Verification items for the finished model (mm, model axes). Face numbers are marked on the shaded views. A direction names the side the tool comes from. Round coordinates to 2 decimals unless told otherwise and drop trailing zeros. Order: outer loops, then holes, each group sorted by start corner. A loop starts at its lowest first (then second) coordinate and runs counter-clockwise, first axis right, second up. Notation, with made-up numbers: (11, 42.25) -> (68, 42.25) arc R32 ccw to (68, 78.25) -> close; hole circle Ø10 at (37.5, 27.25). An arc over 180 degrees is marked (long way). Write item = value, one per line. Start each with the question number.
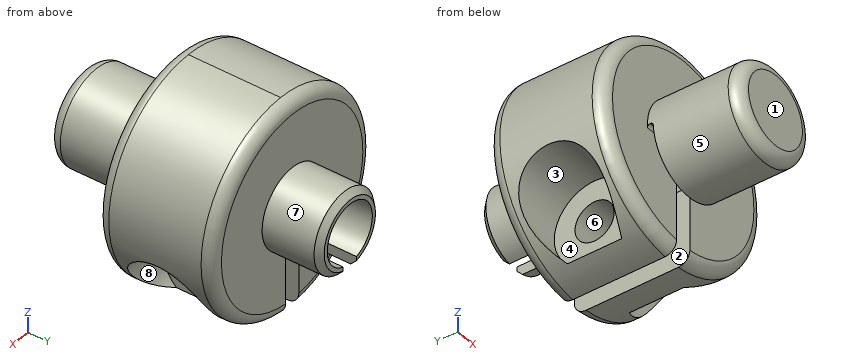
from build123d import *

# Parameters (mm, degrees)
SKETCH1_R            = 4.05
BOSS_EXTRUDE1_DEPTH  = 8
SKETCH2_R            = 9
BOSS_EXTRUDE2_DEPTH  = 10
FILLET1_R            = 1
SKETCH3_R            = 2.55
CUT_EXTRUDE1_DEPTH   = 10
CUT_EXTRUDE2_REACH   = 24.045
M3_CLEARANCE_HOLE1_D = 3.4
SKETCH28_R           = 3.5
CUT_EXTRUDE3_DEPTH   = 6.5
SKETCH29_W           = 8.1
SKETCH29_H           = 0.5
CUT_EXTRUDE7_DEPTH   = 23.045407848
FILLET2_R            = 0.25
BOSS_EXTRUDE3_START  = 5
BOSS_EXTRUDE3_DEPTH  = 5
CHAMFER1_SIZE        = 0.5


with BuildPart() as part:
    # Sketch1 → Boss-Extrude1 (new body)
    with BuildSketch(Plane(origin=(0, 0, 0), x_dir=(1, 0, 0), z_dir=(0, 1, 0))):
        with Locations(Location((0, 0, 0), (0, 0, 270))):
            Circle(SKETCH1_R)
    extrude(amount=BOSS_EXTRUDE1_DEPTH)

    # Sketch2 → Boss-Extrude2 (add)
    with BuildSketch(Plane(origin=(0, 8, 0), x_dir=(1, 0, 0), z_dir=(0, 1, 0))):
        with Locations(Location((0, 0, 0), (0, 0, 270))):
            Circle(SKETCH2_R)
    extrude(amount=BOSS_EXTRUDE2_DEPTH)

    # Fillet1
    fillet1_edges = [part.edges().sort_by_distance(p)[0] for p in [
        (0, 0, -4.05),
        (0, 8, -9),
        (0, 18, -9),
    ]]
    fillet(fillet1_edges, radius=FILLET1_R)

    # Sketch3 → Cut-Extrude1 (cut)
    with BuildSketch(Plane(origin=(0, 18, 0), x_dir=(1, 0, 0), z_dir=(0, 1, 0))):
        with Locations(Location((0, 0, 0), (0, 0, 270))):
            Circle(SKETCH3_R)
    extrude(amount=-CUT_EXTRUDE1_DEPTH, mode=Mode.SUBTRACT)

    # Cut-Extrude2: up to this face of the body (flat: up to its plane)
    cut_extrude2_end = Plane(part.part.faces().sort_by_distance((0, 8, -7.77372583))[0])
    # Sketch20 → Cut-Extrude2 (cut, up to the picked face)
    with BuildSketch(Plane(origin=(0, 18, 0), x_dir=(1, 0, 0), z_dir=(0, 1, 0)), mode=Mode.PRIVATE) as cut_extrude2_sk1:
        with BuildLine():
            Line((-0.75, 2.437211521), (0.75, 2.437211521))
            Line((0.75, 2.437211521), (0.75, 8.968695557))
            ThreePointArc((0.75, 8.968695557), (0, 9), (-0.75, 8.968695557))
            Line((-0.75, 8.968695557), (-0.75, 2.437211521))
        make_face()
    cut_extrude2_tool1 = split(extrude(cut_extrude2_sk1.sketch, amount=-CUT_EXTRUDE2_REACH, mode=Mode.PRIVATE), bisect_by=cut_extrude2_end, keep=Keep.BOTH, mode=Mode.PRIVATE)
    add(cut_extrude2_tool1.solids().sort_by(Axis((0, 18, -5.713399), (0, -1, 0)))[0], mode=Mode.SUBTRACT)

    # M3 Clearance Hole1 (through all)
    with Locations(Plane(origin=(10, 0, 0), x_dir=(0, 0, -1), z_dir=(1, 0, 0))):
        with Locations((5.702953539, 13)):
            Hole(M3_CLEARANCE_HOLE1_D / 2)

    # Sketch28 → Cut-Extrude3 (cut)
    with BuildSketch(Plane(origin=(10, 0, 0), x_dir=(0, 0, -1), z_dir=(1, 0, 0))):
        with Locations((5.702953539, 13)):
            Circle(SKETCH28_R)
    cut_extrude3 = extrude(amount=-CUT_EXTRUDE3_DEPTH, mode=Mode.SUBTRACT)

    # Mirror1: Cut-Extrude3 across plane
    add(cut_extrude3.mirror(Plane(origin=(0, 0, 0), x_dir=(0, 0, 1), z_dir=(1, 0, 0))), mode=Mode.SUBTRACT)

    # Sketch29 → Cut-Extrude7 (cut, through all)
    with BuildSketch(Plane.XY):
        with Locations((0, 7.75)):
            Rectangle(SKETCH29_W, SKETCH29_H)
    extrude(amount=-CUT_EXTRUDE7_DEPTH, mode=Mode.SUBTRACT)

    # Fillet2
    fillet2_edges = [part.edges().sort_by_distance(p)[0] for p in [
        (-3.3, 8, 0),
        (3.3, 8, 0),
        (0, 7.5, 0),
    ]]
    fillet(fillet2_edges, radius=FILLET2_R - 0.0001)  # a hair under: the kernel refuses the full size

    # Sketch30 → Boss-Extrude3 (add)
    with BuildSketch(Plane(origin=(0, 18, 0), x_dir=(1, 0, 0), z_dir=(0, 1, 0)).offset(BOSS_EXTRUDE3_START)):
        with BuildLine():
            Line((-0.75, 3.31624788), (-0.75, 2.437211521))
            ThreePointArc((-0.75, 2.437211521), (0, -2.55), (0.75, 2.437211521))
            Line((0.75, 2.437211521), (0.75, 3.31624788))
            ThreePointArc((0.75, 3.31624788), (0, -3.4), (-0.75, 3.31624788))
        make_face()
    extrude(amount=-BOSS_EXTRUDE3_DEPTH)

    # Chamfer1
    chamfer1_edges = [part.edges().sort_by_distance(p)[0] for p in [
        (0, 23, 3.4),
    ]]
    chamfer(chamfer1_edges, length=CHAMFER1_SIZE)


solid = part.part
(1) Cross-section at B-B (x = 1.5). Give the number of separate pieces and of enclosed holes in the cut face, and give its area (3 significant figures).
(2) Draft check along Y on the marked faces 1, 2 and 3. Enter one of: +Y half, -Y half, draft (parallel to the pull), parting line (faces both ways), or undercut.
(3) Cross-section at D-D (y = 4). Enter the section's corners in (x, z).
(4) Depth check by flat-ended pin: pin 1 (6 mm diameter, centred on x = -5.5, y = 4.5, fed in from -Z); pin 2 (5.5 mm diameter, centred on y = 13, z = -5.7, fed in from +X); pin 3 (3 mm diameter, centred on y = 12, z = -5, fed in from -X). Enter the tip coordinate at first touch or a pass-through.
(5) Scan lines: line 1 along X through (y, z) = (13, 0); line 2 along X through (y, z) = (20.2, 0); line 3 along Z through (x, y) = (0, 21). Record each from-to range of solid material in increasing order. Write a range as from..to.
(6) Cross-section at A-A (y = 13). Enter the section's corners in (x, z), and give its area (3 significant figures).
(7) Set-up check for the marked faces 4, 5, 6, 7 and 8: record each of +Z, -Z, +X, -X, +Y, -Y from which the full face is reachable in a straight line by a thin tool's end or side.
Outcome:
q1.separate_pieces = 2
q1.enclosed_holes = 1
q1.area = 194 mm^2
q2.face_1 = -Y half
q2.face_2 = draft
q2.face_3 = undercut
q3.outline = circle Ø8.1 at (0, 0)
q4.pin_1 = -3.19
q4.pin_2 = 3.5
q4.pin_3 = -3.5
q5.line_1 = -9..-2.55, 2.55..9
q5.line_2 = -3.4..-2.55, 2.55..3.4
q5.line_3 = 2.55..3.4
q6.outline = (-8.73, -2.2) -> (-3.5, -2.2) -> (-3.5, -4) -> (-0.75, -4) -> (-0.75, -2.44) arc R2.55 cw (long way) to (0.75, -2.44) -> (0.75, -4) -> (3.5, -4) -> (3.5, -2.2) -> (8.73, -2.2) arc R9 ccw (long way) to start; (-3.5, -8.29) arc R9 ccw to (-0.75, -8.97) -> (-0.75, -7.4) -> (-3.5, -7.4) -> close; (0.75, -8.97) arc R9 ccw to (3.5, -8.29) -> (3.5, -7.4) -> (0.75, -7.4) -> close
q6.area = 164 mm^2
q7.face_4 = -X
q7.face_5 = -Y
q7.face_6 = +X, -X
q7.face_7 = +Y
q7.face_8 = +X
